from build123d import *

# Parameters (mm, degrees)
BOSS_EXTRUDE1_DEPTH = 10
BOSS_EXTRUDE2_DEPTH = 2


with BuildPart() as part:
    # Sketch3 → Boss-Extrude1 (new body)
    with BuildSketch(Plane(origin=(0, 0, 0), x_dir=(1, 0, 0), z_dir=(0, 1, 0))):
        Polygon((19.916769016, 5.321871098), (19.997399332, 0.322521265), (0, 0), (-17.156995198, -10.278011275), (-19.726498017, -5.988762475), (-1.420202067, 4.977745005), align=None)
    extrude(amount=BOSS_EXTRUDE1_DEPTH)

    # Sketch4 → Boss-Extrude2 (add)
    with BuildSketch(Plane(origin=(0, 10, 0), x_dir=(1, 0, 0), z_dir=(0, 1, 0))):
        Polygon((-19.726498017, -5.988762475), (-17.156995198, -10.278011275), (-11.166429161, -20.278011275), (20.158680936, -9.677478735), (19.997399332, 0.322521265), (19.916769016, 5.321871098), (-1.420202067, 4.977745005), align=None)
    boss_extrude2 = extrude(amount=BOSS_EXTRUDE2_DEPTH)

    # Mirror1: Boss-Extrude2 across plane
    add(boss_extrude2.mirror(Plane.ZX.offset(5)))


solid = part.part
Input: part model. Units: mm. Frame: model coordinates. A direction names the side the tool comes from. Round coordinates to 2 decimals unless told otherwise and drop trailing zeros. Loops run counter-clockwise (first coordinate to the right, second up) from the corner with the lowest first, then second, coordinate; pieces in that order, holes last. Notation, with made-up numbers: (18, 45.25) -> (39, 45.25) arc R11 cw to (39, 52.25) -> close; hole circle Ø3 at (89.25, -29). An arc over 180 degrees is marked (long way). Answer as a JSON object with one key per item and string values. Group by question number.
1) Pin query (flat end, axial travel): pin 1 (1 mm diameter, centred on y = 0, z = 7, fed in from -X); pin 2 (6 mm diameter, centred on x = 9, y = 9, fed in from +Z); pin 3 (2 mm diameter, centred on x = 6.5, y = 5, fed in from -Z). Return the tip coordinate at first contact, or that it passes through.
2) Reachability of faces 5 (the flat face through (1, 0, 8)), 6 (the flat face through (4.28, 10.99, 15.05)) from +Z, -Z, +X, -X, +Y, -Y: full face, straight path, thin tool, end or side. Return the list, or none.
3) Section query B-B on x = -7.5. Output: boundary loops of the cut face in (y, z), plus the area to 3 significant figures.
4) Section query D-D on z = 1.5. Output: boundary loops of the cut face in (x, y), plus the area to 3 significant figures.
5) Section query C-C on y = 3. Output: boundary loops of the cut face in (x, z).
6) Draft query along Y for faces 1 (the flat face through (-8.46, 4.93, 5.07)), 2 (the flat face through (0, -2, 7)), 3 (the flat face through (1, 10, 8)), 4 (the flat face through (-10.4, 5.1, 0.4)). Return one class per face: +Y half, -Y half, draft (parallel to the pull), parting line (faces both ways), or undercut.
7) Section query A-A on z = 16.25. Output: boundary loops of the cut face in (x, y).
8) Ray query, L1, parallel to Y at x = 18.5, z = 3.5; L2, parallel to Z at x = -13, y = 5; L3, parallel to X at y = 6, z = -0.5. Return the intervals inside material, ascending.
Reply:
{
 "1": {"pin 1": "stops at x = -19.42", "pin 2": "stops at z = 14.41", "pin 3": "stops at z = -5.12"},
 "2": {"face 5": "+Z, +X", "face 6": "+Z, +X, +Y, -Y"},
 "3": {"outline": "(-2, -1.34) -> (12, -1.34) -> (12, 19.04) -> (10, 19.04) -> (10, 4.49) -> (0, 4.49) -> (0, 19.04) -> (-2, 19.04) -> close", "area": "140 mm2"},
 "4": {"outline": "(-12.23, -2) -> (20.03, -2) -> (20.03, 0) -> (-2.5, 0) -> (-2.5, 10) -> (20.03, 10) -> (20.03, 12) -> (-12.23, 12) -> close", "area": "226 mm2"},
 "5": {"outline": "(-19.73, 5.99) -> (-1.42, -4.98) -> (19.92, -5.32) -> (20, -0.32) -> (0, 0) -> (-17.16, 10.28) -> close"},
 "6": {"face 1": "undercut", "face 2": "-Y half", "face 3": "undercut", "face 4": "draft"},
 "7": {"outline": "(-13.58, -2) -> (0.74, -2) -> (0.74, 0) -> (-13.58, 0) -> close; (-13.58, 10) -> (0.74, 10) -> (0.74, 12) -> (-13.58, 12) -> close"},
 "8": {"L1": "y = -2 to 0, 10 to 12", "L2": "z = 1.96 to 7.79", "L3": "x = -8.89 to 19.99"}
}
